Read the model definition and answer for the solid it produces. Units are mm, in the model's axes. Round coordinates to 2 decimals unless told otherwise and drop trailing zeros. Order: outer loops, then holes, each group sorted by start corner. A loop starts at its lowest first (then second) coordinate and runs counter-clockwise, first axis right, second up.
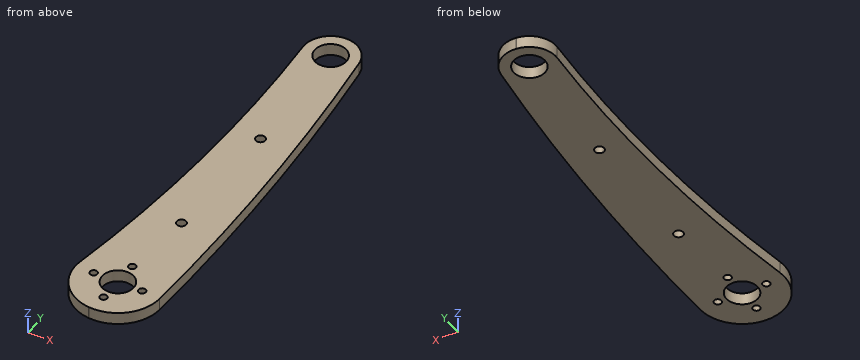
from build123d import *

# Parameters (mm, degrees)
SKETCH_1_R          = 1.925
SKETCH_1_R_2        = 0.925
SKETCH_1_R_3        = 6.5
EXTRUDE_1_DEPTH     = 5
SKETCH_2_R          = 1.5
CUT_EXTRUDE_1_DEPTH = 161.109426861


with BuildPart() as part:
    # 草图1 → 凸台-拉伸1 (new body)
    with BuildSketch(Plane.XY):
        with BuildLine():
            Line((-1.197146646, 158.934662313), (-0.998147001, 158.954620147))
            ThreePointArc((-0.998147001, 158.954620147), (6.901917658, 156.565251464), (10.916367847, 149.353851183))
            ThreePointArc((10.916367847, 149.353851183), (17.20705989, 74.502805076), (17.564366606, -0.61126978))
            ThreePointArc((17.564366606, -0.61126978), (11.601405763, -13.20181841), (-1.651060868, -17.497274731))
            Line((-1.651060868, -17.497274731), (-1.850065436, -17.477353429))
            ThreePointArc((-1.850065436, -17.477353429), (-13.988103687, -10.64018704), (-17.337003373, 2.882523033))
            ThreePointArc((-17.337003373, 2.882523033), (-9.795741354, 74.828468127), (-10.96780908, 147.159069574))
            ThreePointArc((-10.96780908, 147.159069574), (-8.465381447, 155.024052744), (-1.197146646, 158.934662313))
        make_face()
        with Locations((2.5, 40)):
            Circle(SKETCH_1_R, mode=Mode.SUBTRACT)
        with Locations((2.5, 95)):
            Circle(SKETCH_1_R, mode=Mode.SUBTRACT)
        with Locations((10, 0)):
            Circle(SKETCH_1_R_2, mode=Mode.SUBTRACT)
        with Locations((0, -10)):
            Circle(SKETCH_1_R_2, mode=Mode.SUBTRACT)
        with Locations((0, 10)):
            Circle(SKETCH_1_R_2, mode=Mode.SUBTRACT)
        with Locations((-10, 0)):
            Circle(SKETCH_1_R_2, mode=Mode.SUBTRACT)
        Circle(SKETCH_1_R_3, mode=Mode.SUBTRACT)
        with Locations((0, 148)):
            Circle(SKETCH_1_R_3, mode=Mode.SUBTRACT)
    extrude(amount=EXTRUDE_1_DEPTH)

    # 草图2 → 切除-拉伸1 (cut, through all)
    with BuildSketch(Plane.XY.offset(5)):
        with Locations((0, 10)):
            Circle(SKETCH_2_R)
        with Locations((10, 0)):
            Circle(SKETCH_2_R)
        with Locations((-10, 0)):
            Circle(SKETCH_2_R)
        with Locations((0, -10)):
            Circle(SKETCH_2_R)
    extrude(amount=-CUT_EXTRUDE_1_DEPTH, mode=Mode.SUBTRACT)


solid = part.part
Q1. Straight lines are drawn through the part: probe 1 along Y at (x, z) = (0, 2.3) (3 decimals); probe 2 along Y at (x, z) = (-3, 4.75); probe 3 along X at (y, z) = (95, 2.85) (3 decimals). For each, find the intervals that lie inside material, in ascending order.
Outcome:
probe 1: y = -17.575 to -11.5, -8.5 to -6.5, 6.5 to 8.5, 11.5 to 141.5, 154.5 to 159
probe 2: y = -17.32 to -5.77, 5.77 to 142.23, 153.77 to 158.58
probe 3: x = -9.245 to 0.575, 4.425 to 16.076
Q2. A cutting plane is placed at B-B, the plane z = 2.25. Give the number of separate pieces and of enclosed holes in the cut face, plus the area to 3 significant figures.
Outcome:
separate pieces: 1
enclosed holes: 8
area: 4,450 mm2
Q3. A cutting plane is placed at A-A, the plane y = 95. Give the vertices of the cut face in (x, z) (3 decimals), plus the area to 3 significant figures.
Outcome:
outline: (-9.245, 0) - (0.575, 0) - (0.575, 5) - (-9.245, 5) - close; (4.425, 0) - (16.076, 0) - (16.076, 5) - (4.425, 5) - close
area: 107 mm2
Q4. A cutting plane is placed at D-D, the plane y = 115. Give the vertices of the cut face in (x, z).
Outcome:
outline: (-9.37, 0) - (14.54, 0) - (14.54, 5) - (-9.37, 5) - close
Q5. Flat-ended cylindrical pins translate along their axes: pin 1 (1.5 mm diameter, centred on y = 129.5, z = 2, fed in from +X); pin 2 (1.5 mm diameter, centred on x = 3, z = 4, fed in from -Y). Find the tip coordinate at first contact, or state that the pin passes through.
Outcome:
pin 1: stops at x = 13.24
pin 2: stops at y = -17.43
Q6. A cutting plane is placed at C-C, the plane y = 40. Give the vertices of the cut face in (x, z) (3 decimals).
Outcome:
outline: (-12.351, 0) - (0.575, 0) - (0.575, 5) - (-12.351, 5) - close; (4.425, 0) - (18.109, 0) - (18.109, 5) - (4.425, 5) - close
